from build123d import *

# Parameters (mm, degrees)
SKETCH_R           = 12.25
SKETCH_R_2         = 2
PAD_DEPTH          = 3
SKETCH001_R        = 12.25
SKETCH001_R_2      = 10.5
PAD001_DEPTH       = 30
PAD002_DEPTH       = 3
POLARPATTERN_COUNT = 2
PAD003_DEPTH       = 23
CHAMFER_SIZE       = 2


with BuildPart() as part:
    # Sketch → Pad (new body)
    with BuildSketch(Plane.XY):
        Circle(SKETCH_R)
        Circle(SKETCH_R_2, mode=Mode.SUBTRACT)
    extrude(amount=-PAD_DEPTH)

    # Sketch001 → Pad001 (join)
    with BuildSketch(Plane.XY):
        Circle(SKETCH001_R)
        Circle(SKETCH001_R_2, mode=Mode.SUBTRACT)
    extrude(amount=PAD001_DEPTH)

    # Sketch002 → Pad002 (join)
    with BuildSketch(Plane.XY.offset(30)):
        with BuildLine():
            ThreePointArc((0, 7.75), (-5.480078, 5.480078), (-7.75, 0))
            Line((-12.25, 0), (-7.75, 0))
            ThreePointArc((0, 12.25), (-8.662058, 8.662058), (-12.25, 0))
            Line((0, 7.75), (0, 12.25))
        make_face()
    pad002 = extrude(amount=-PAD002_DEPTH)

    # PolarPattern: Pad002 ×2 about axis
    polarpattern_axis = Axis((0, 0, 30), (0, 0, 1))
    for i in range(1, POLARPATTERN_COUNT):
        add(pad002.rotate(polarpattern_axis, i * 360 / POLARPATTERN_COUNT))

    # Sketch003 (on DatumPlane) → Pad003 (join)
    with BuildSketch(Plane.XY.offset(23)):
        with BuildLine():
            ThreePointArc((-3.170533, 11.832591), (-8.662058, 8.662058), (-11.832591, 3.170533))
            Line((-7.485925, 2.005848), (-11.832591, 3.170533))
            ThreePointArc((-2.005848, 7.485925), (-5.480078, 5.480078), (-7.485925, 2.005848))
            Line((-3.170533, 11.832591), (-2.005848, 7.485925))
        make_face()
    extrude(amount=-PAD003_DEPTH)

    # Chamfer
    chamfer_edges = [part.edges().sort_by_distance(p)[0] for p in [
        (-2, 0, -3),
    ]]
    chamfer(chamfer_edges, length=CHAMFER_SIZE)


solid = part.part
Input: part model. Units: mm. Frame: model coordinates. A direction names the side the tool comes from. Coordinates: 2 decimals unless noted, no trailing zeros. Loops run counter-clockwise (first coordinate to the right, second up) from the corner with the lowest first, then second, coordinate; pieces in that order, holes last.
Q1. Cut plane A-A (z = 22). Output: boundary loops of the cut face in (x, y).
Q2. Draft query along X for faces 4 (the face through (-3, 3, -3)), 5 (the face through (-8.8, 2.36, 11.66)). Return one class per face: +X half, -X half, draft (parallel to the pull), parting line (faces both ways), or undercut.
Q3. Set-up query: faces 1 (the face through (-6, 6, 23)), 2 (the face through (-5.42, 5.54, 28.52)), 3 (the face through (-0.434, -1.952, -0.493)). Return all of +Z, -Z, +X, -X, +Y, -Y with unobstructed straight access to the full face (end or side cutting, diameter ignored); none if empty.
Q4. Contact query for flat-ended pins moving along their axis: pin 1 (1.4 mm diameter, centred on y = 8.5, z = 29, fed in from +X); pin 2 (10 mm diameter, centred on y = -7.5, z = 5, fed in from +X); pin 3 (2 mm diameter, centred on x = 9, z = 29, fed in from +Y); pin 4 (1.5 mm diameter, centred on x = -1, y = 0, fed in from -Z). Output: stop coordinate, or through.
Q5. Cut plane C-C (z = 26). Output: boundary loops of the cut face in (x, y).
Q6. Cut plane B-B (y = 7). Output: boundary loops of the cut face in (x, z), then the cut area to 3 significant figures.
Q7. Cut plane D-D (y = 9.5). Output: boundary loops of the cut face in (x, z), then the cut area to 3 significant figures.
Q8. Material intervals for line 1 (Z direction, x = 6.25, y = -5.25); line 2 (Y direction, x = 0, z = -0.3); line 3 (Y direction, x = 0, z = 10.5), sorted ascending.
Working result:
1. outline: circle Ø24.5 at (0, 0); hole (-10.14, 2.72) arc R10.5 ccw (long way) to (-2.72, 10.14) - (-2.01, 7.49) arc R7.75 ccw to (-7.49, 2.01) - close
2. face 4: draft
2. face 5: undercut
3. face 1: none
3. face 2: +Z
3. face 3: +Z, -Z
4. pin 1: stops at x = 9.45
4. pin 2: stops at x = 11.99
4. pin 3: stops at y = 9.28
4. pin 4: passes through
5. outline: circle Ø24.5 at (0, 0); hole circle Ø21 at (0, 0)
6. outline: (-10.05, -3) - (10.05, -3) - (10.05, 30) - (7.83, 30) - (7.83, 0) - (-3.33, 0) - (-3.33, 23) - (-7.83, 23) - (-7.83, 27) - (-3.33, 27) - (-3.33, 30) - (-10.05, 30) - close
6. area: 311 mm2
7. outline: (-7.73, -3) - (7.73, -3) - (7.73, 30) - (4.47, 30) - (4.47, 0) - (-2.55, 0) - (-2.55, 23) - (-4.47, 23) - (-4.47, 27) - (0, 27) - (0, 30) - (-7.73, 30) - close
7. area: 300 mm2
8. line 1: z = -3 to 0, 27 to 30
8. line 2: y = -12.25 to -2, 2 to 12.25
8. line 3: y = -12.25 to -10.5, 10.5 to 12.25
